Could you check a few things on this model? Use its own coordinates, in mm. Face numbers are marked on the shaded views. A direction names the side the tool comes from. Round coordinates to 2 decimals unless told otherwise and drop trailing zeros. Loops run counter-clockwise (first coordinate to the right, second up) from the corner with the lowest first, then second, coordinate; pieces in that order, holes last. Notation, with made-up numbers: (7, 55.25) -> (47, 55.25) arc R8 ccw to (47, 66.25) -> close; hole circle Ø7 at (56.25, 43.5). An arc over 180 degrees is marked (long way). One line per item, written item: value.
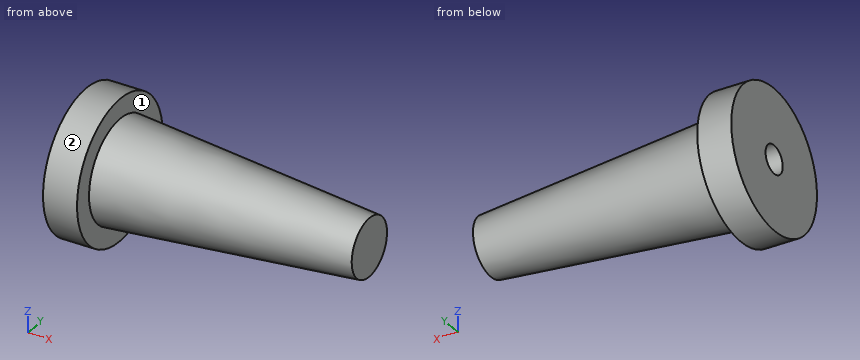
from build123d import *

# Parameters (mm, degrees)
SKETCH_9_R          = 5
CUT_EXTRUDE_2_DEPTH = 30
MM_1_D              = 4
MM_1_DEPTH          = 6
MM_1_TIP            = 1.201721238


with BuildPart() as part:
    # 草图5 → 旋转1 (revolve)
    with BuildSketch(Plane.XY, mode=Mode.PRIVATE) as revolve_1_sk:
        Polygon((-50, 0), (-50, 25), (-38, 25), (-38, 18), (50, 10.30099761), (50, 0), align=None)
    revolve(revolve_1_sk.sketch.rotate(Axis((-110.009795311, 0, 0), (1, 0, 0)), 90), axis=Axis((-110.009795311, 0, 0), (1, 0, 0)))

    # 草图9 → 切除-拉伸2 (cut)
    with BuildSketch(Plane.ZY.offset(50)):
        Circle(SKETCH_9_R)
    extrude(amount=-CUT_EXTRUDE_2_DEPTH, mode=Mode.SUBTRACT)

    # 大小mm 暗销孔1
    with Locations(Plane.ZY.offset(20)):
        with Locations((0, 0)):
            Hole(MM_1_D / 2, depth=MM_1_DEPTH)
            with Locations((0, 0, -(MM_1_DEPTH + MM_1_TIP / 2))):  # 118° drill point
                Cone(0, MM_1_D / 2, MM_1_TIP, mode=Mode.SUBTRACT)


solid = part.part
(1) If we section it at D-D, the plane z = -21: Please give me the cut outline in (x, y).
Recorded:
outline: (-50, -13.56) -> (-38, -13.56) -> (-38, 13.56) -> (-50, 13.56) -> close
(2) If I drill on L1, parallel to X at y = -4.5, z = -18.5; L2, parallel to Y at x = -43.25, z = 0; L3, parallel to Y at x = -35.5, z = -1, over which ranges is the centre line in solid material (lowest first)?
Recorded:
L1: -50 to -38
L2: -25 to -5, 5 to 25
L3: -17.75 to -4.9, 4.9 to 17.75
(3) If we section it at C-C, the plane x = 27: Please give me the cut outline in (y, z), then the cut area to 3 significant figures.
Recorded:
outline: circle Ø24.63 at (0, 0)
area: 476 mm²
(4) I'm going to push flat-ended pins straight in: pin 1 Ø4 at (y, z) = (13.5, 17.5) entering from +X; pin 2 Ø5 at (x, y) = (36, 4) entering from +Z; pin 3 Ø10 at (x, z) = (36.5, -11.5) entering from -Y. Where does each tip first touch, or does it pass through?
Recorded:
pin 1: x = -38
pin 2: z = 11.49
pin 3: y = -9.51
(5) If we section it at B-B, the plane z = 19: Please give me the cut outline in (x, y), then the cut area to 3 significant figures.
Recorded:
outline: (-50, -16.25) -> (-38, -16.25) -> (-38, 16.25) -> (-50, 16.25) -> close
area: 390 mm²
(6) If we section it at A-A, the plane x = -26: Please give me the cut outline in (y, z), then the cut area to 3 significant figures.
Recorded:
outline: circle Ø33.9 at (0, 0); hole circle Ø10 at (0, 0)
area: 824 mm²
(7) For the marked faces 1 and 2, which set-ups out of +Z, -Z, +X, -X, +Y, -Y let a thin tool reach every point of the face, with its end or its side?
Recorded:
face 1: +X
face 2: +X, -X
